Here's how the part is built. I have some questions about the finished solid (model axes, mm). Face numbers are marked on the shaded views. A direction names the side the tool comes from. Round coordinates to 2 decimals unless told otherwise and drop trailing zeros. Order: outer loops, then holes, each group sorted by start corner. A loop starts at its lowest first (then second) coordinate and runs counter-clockwise, first axis right, second up. Notation, with made-up numbers: (19.5, -2.5) - (27.5, -2.5) arc R26 cw to (27.5, 23.5) - close; hole circle Ø3 at (43, -14.75). An arc over 180 degrees is marked (long way). One line per item, written item: value.
from build123d import *

# Parameters (mm, degrees)
F0_W     = 500
F0_H     = 18
F1_DEPTH = 115
F2_W     = 220
F2_H     = 92
F3_DEPTH = 275
F4_R     = 5
F5_W     = 387.605816
F5_H     = 94.405166
F6_DEPTH = 120.001


with BuildPart() as f1:
    # F0 (on Front) → F1 (new body, symmetric)
    with BuildSketch(Plane.XZ):
        Rectangle(F0_W, F0_H)
        Polygon((-250, -111), (-250, -9), (-250, 9), (-268, 9), (-268, -111), align=None)
        Polygon((250, 9), (250, -9), (250, -111), (268, -111), (268, 9), align=None)
    extrude(amount=F1_DEPTH, both=True)

    # F2 (on Right) → F3 (cut, symmetric)
    with BuildSketch(Plane.YZ):
        with Locations((0, -60)):
            Rectangle(F2_W, F2_H)
    extrude(amount=F3_DEPTH, both=True, mode=Mode.SUBTRACT)

    # F4
    f4_edges = [f1.edges().sort_by_distance(p)[0] for p in [
        (259, 115, -111),
        (-259, 115, -111),
        (-259, -115, -111),
        (259, -115, -111),
        (0, -115, 9),
        (0, 115, 9),
        (-268, 0, 9),
        (268, 0, 9),
    ]]
    fillet(f4_edges, radius=F4_R)

    # F5 (on face) → F6 (cut, through all)
    with BuildSketch(Plane.XY.offset(9)):
        Rectangle(F5_W, F5_H)
    extrude(amount=-F6_DEPTH, mode=Mode.SUBTRACT)


solid = f1.part
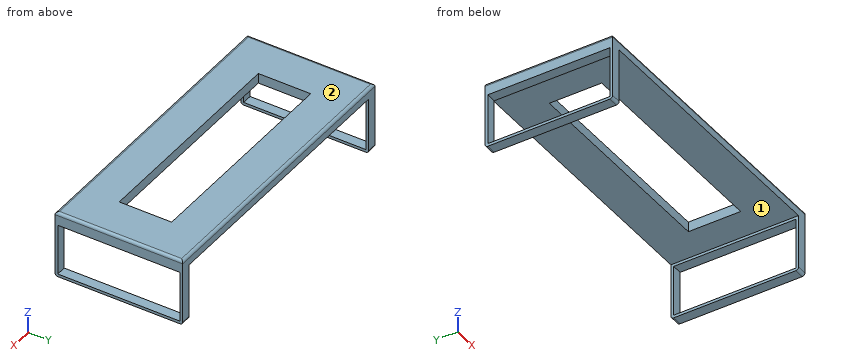
Q1. If we section it at B-B, the plane z = -1.5: Please give me the cut outline in (x, y).
Results list:
outline: (-268, -115) - (268, -115) - (268, 115) - (-268, 115) - close; hole (-193.8, -47.2) - (193.8, -47.2) - (193.8, 47.2) - (-193.8, 47.2) - close
Q2. If we section it at C-C, the plane x = -15: Please give me the cut outline in (y, z).
Results list:
outline: (-115, -9) - (-47.2, -9) - (-47.2, 9) - (-110, 9) arc R5 ccw to (-115, 4) - close; (47.2, -9) - (115, -9) - (115, 4) arc R5 ccw to (110, 9) - (47.2, 9) - close
Q3. Which directions (+Z, -Z, +X, -X, +Y, -Y) give clear straight access to the entire face, cutting with the end or side of a thin tool? Please do the marked faces 1 and 2.
Results list:
face 1: -Z, +Y, -Y
face 2: +Z, +X, -X, +Y, -Y
Q4. Will this pin go through, and if not, where does the flat tip stop? pin 1 (2 mm diameter, centred on x = -96, y = 75.5, fed in from -Z).
Results list:
pin 1: z = -9
Q5. If we section it at D-D, the plane z = -67.5: Please give me the cut outline in (x, y), then the cut area to 3 significant figures.
Results list:
outline: (-268, -115) - (-250, -115) - (-250, -110) - (-268, -110) - close; (-268, 110) - (-250, 110) - (-250, 115) - (-268, 115) - close; (250, -115) - (268, -115) - (268, -110) - (250, -110) - close; (250, 110) - (268, 110) - (268, 115) - (250, 115) - close
area: 360 mm²
Q6. If I drill on line 1 along X through (y, z) = (-33, 3); line 2 along Z through (x, y) = (240.5, 101), over which ranges is the centre line in solid material (lowest first)?
Results list:
line 1: -268 to -193.8, 193.8 to 268
line 2: -9 to 9
Q7. If we section it at A-A, the plane y = -84.5: Please give me the cut outline in (x, z).
Results list:
outline: (-268, -111) - (-250, -111) - (-250, -106) - (-268, -106) - close; (-268, -14) - (-250, -14) - (-250, -9) - (250, -9) - (250, -14) - (268, -14) - (268, 4) arc R5 ccw to (263, 9) - (-263, 9) arc R5 ccw to (-268, 4) - close; (250, -111) - (268, -111) - (268, -106) - (250, -106) - close
